```python
from build123d import *

# Parameters (mm, degrees)
SKETCH_1_W          = 19.1
SKETCH_1_H          = 20.55
EXTRUDE_1_DEPTH     = 1.2
SKETCH_2_W          = 1.844375839
SKETCH_2_H          = 10
EXTRUDE_2_DEPTH     = 8.7
SKETCH_3_W          = 7.5
SKETCH_3_H          = 5
EXTRUDE_3_DEPTH     = 8.7
SKETCH_4_W          = 8
SKETCH_4_H          = 7.55
EXTRUDE_4_DEPTH     = 11
SKETCH_5_W          = 10.3
SKETCH_5_H          = 4
EXTRUDE_5_DEPTH     = 4.5
SKETCH_6_R          = 0.5
CUT_EXTRUDE_1_DEPTH = 18.826332349


with BuildPart() as part:
    # ｽｹｯﾁ1 → ﾎﾞｽ - 押し出し1 (new body)
    with BuildSketch(Plane.XY):
        Rectangle(SKETCH_1_W, SKETCH_1_H)
    extrude(amount=EXTRUDE_1_DEPTH)

    # ｽｹｯﾁ2 → ﾎﾞｽ - 押し出し2 (add)
    with BuildSketch(Plane.XY.offset(1.2)):
        with Locations((7.877812081, 5.275)):
            Rectangle(SKETCH_2_W, SKETCH_2_H)
    extrude_2 = extrude(amount=EXTRUDE_2_DEPTH)

    # ﾐﾗｰ1: ﾎﾞｽ - 押し出し2 across plane
    add(extrude_2.mirror(Plane(origin=(0, 0, 0), x_dir=(0, 0, 1), z_dir=(1, 0, 0))))

    # ｽｹｯﾁ3 → ﾎﾞｽ - 押し出し3 (add)
    with BuildSketch(Plane(origin=(0, 0, 0), x_dir=(-1, 0, 0), z_dir=(0, 0, -1))):
        with Locations((-5.05, -2.475)):
            Rectangle(SKETCH_3_W, SKETCH_3_H)
    extrude(amount=EXTRUDE_3_DEPTH)

    # ｽｹｯﾁ4 → ﾎﾞｽ - 押し出し4 (add)
    with BuildSketch(Plane(origin=(0, 0, 0), x_dir=(-1, 0, 0), z_dir=(0, 0, -1))):
        with Locations((4.7, -5.3)):
            Rectangle(SKETCH_4_W, SKETCH_4_H)
    extrude(amount=EXTRUDE_4_DEPTH)

    # ｽｹｯﾁ5 → ﾎﾞｽ - 押し出し5 (add)
    with BuildSketch(Plane(origin=(0, 0, 0), x_dir=(-1, 0, 0), z_dir=(0, 0, -1))):
        with Locations((-0.7, 7.975)):
            Rectangle(SKETCH_5_W, SKETCH_5_H)
    extrude(amount=EXTRUDE_5_DEPTH)

    # ｽｹｯﾁ6 → ｶｯﾄ - 押し出し1 (cut, through all)
    with BuildSketch(Plane(origin=(0, 0, 0), x_dir=(-1, 0, 0), z_dir=(0, 0, -1))):
        with Locations((-5.35, -6.775)):
            Circle(SKETCH_6_R)
        with Locations((-5.35, -9.315)):
            Circle(SKETCH_6_R)
    extrude(amount=-CUT_EXTRUDE_1_DEPTH, mode=Mode.SUBTRACT)


solid = part.part
```
For this review, take the finished solid that the model builds, in its own axes (mm). A direction names the side the tool comes from. Give positions to 0.01 mm unless a question says otherwise; leave off trailing zeros. Write each loop counter-clockwise with the first axis right and the second up, starting at its lowest first coordinate (ties: lowest second). Pieces come first, ordered by that corner, then holes.
Item 1: Wall thickness on probe 1 along Y at (x, z) = (5.35, 0.75) (3 decimals); probe 2 along X at (y, z) = (-2.5, -2); probe 3 along X at (y, z) = (9.25, 2): over which ranges is each line inside the solid? List them lowest first.
Item 2: Machinability: for faces 4 (the face through (1, 8, -4.5)), 5 (the face through (5, -4.975, -4)), 6 (the face through (-6.956, 5, 5)), which of the approach directions +Z, -Z, +X, -X, +Y, -Y give a long, thin tool a straight path to every point of the face, cutting with its end or side? Answer none if there is none.
Item 3: The part is to be moulded in two halves that separate along Y. For faces 1 (the face through (-5, -9.075, -5)), 2 (the face through (1, 5.975, -2)), 3 (the face through (9.55, 0, 1)), say which applies: +Y half, -Y half, draft (parallel to the pull), parting line (faces both ways), or undercut.
Item 4: Take a section at B-B (z = 5). Give the boundary of the cut face in (x, y) (3 decimals).
Item 5: Take a section at C-C (y = 4.75). Give the boundary of the cut face in (x, z), and give its area (3 significant figures).
Item 6: Take a section at D-D (z = -0.75). Give the boundary of the cut face in (x, y) (3 decimals), and give its area (3 significant figures).
Item 7: Take a section at A-A (x = 5.35). Give the boundary of the cut face in (y, z) (3 decimals), and give its area (3 significant figures).
Item 8: Insertion check: P1, Ø1, axis at x = 3, y = 6.5, coming from the +Z side; P2, Ø3.5, axis at x = -1.5, z = -2, coming from the +Y side (3 decimals); P3, Ø1.5, axis at x = 8, z = 6.5, coming from the -Y side (3 decimals); P4, Ø6, axis at x = 0.5, z = 5.5, coming from the -Y side (3 decimals). Each pin has a flat end and moves straight along its axis. Give the tip position at first contact, or say it passes through.
Established:
1. probe 1: y = -10.275 to -9.815, -8.815 to -7.275, -6.275 to 10.275
1. probe 2: x = -8.7 to -0.7, 1.3 to 8.8
1. probe 3: x = -8.8 to -6.96, 6.96 to 8.8
2. face 4: -Z, +X, -X, +Y
2. face 5: -Z, +X, -Y
2. face 6: +Z, +Y, -Y
3. face 1: -Y half
3. face 2: undercut
3. face 3: draft
4. outline: (-8.8, 0.275) - (-6.956, 0.275) - (-6.956, 10.275) - (-8.8, 10.275) - close; (6.956, 0.275) - (8.8, 0.275) - (8.8, 10.275) - (6.956, 10.275) - close
5. outline: (-9.55, 0) - (9.55, 0) - (9.55, 1.2) - (8.8, 1.2) - (8.8, 9.9) - (6.96, 9.9) - (6.96, 1.2) - (-6.96, 1.2) - (-6.96, 9.9) - (-8.8, 9.9) - (-8.8, 1.2) - (-9.55, 1.2) - close
5. area: 55.0 mm2
6. outline: (-8.7, -9.075) - (-0.7, -9.075) - (-0.7, -1.525) - (-8.7, -1.525) - close; (-4.45, 5.975) - (5.85, 5.975) - (5.85, 9.975) - (-4.45, 9.975) - close; (1.3, -4.975) - (8.8, -4.975) - (8.8, 0.025) - (1.3, 0.025) - close
6. area: 139 mm2
7. outline: (-10.275, 0) - (-9.815, 0) - (-9.815, 1.2) - (-10.275, 1.2) - close; (-8.815, 0) - (-7.275, 0) - (-7.275, 1.2) - (-8.815, 1.2) - close; (-6.275, 0) - (-4.975, 0) - (-4.975, -8.7) - (0.025, -8.7) - (0.025, 0) - (5.975, 0) - (5.975, -4.5) - (9.975, -4.5) - (9.975, 0) - (10.275, 0) - (10.275, 1.2) - (-6.275, 1.2) - close
7. area: 83.8 mm2
8. P1: stops at z = 1.2
8. P2: stops at y = 9.975
8. P3: stops at y = 0.275
8. P4: passes through
